Could you check a few things on this model? Use its own coordinates, in mm. A direction names the side the tool comes from. Round coordinates to 2 decimals unless told otherwise and drop trailing zeros. Write each loop counter-clockwise with the first axis right and the second up, starting at its lowest first coordinate (ties: lowest second). Pieces come first, ordered by that corner, then holes. Notation, with made-up numbers: (34, -25.75) -> (73, -25.75) arc R14 cw to (73, -13.75) -> close; hole circle Ø3 at (24, 52.25). An arc over 180 degrees is marked (long way). One line per question, with ' | ' between items. Start each with the question number.
1. For faces 4 (the flat face through (16, -3, 10)), 5 (the flat face through (0, 0, -8)), 6 (the flat face through (0, 0, 5)), 7 (the cylindrical face through (-0.29, 2.23, -3.94)), which set-ups out of +Z, -Z, +X, -X, +Y, -Y let a thin tool reach every point of the face, with its end or its side?
2. If I drill on line 1 along Y through (x, z) = (21.75, 25); line 2 along X through (y, z) = (-4, 27); line 3 along Z through (x, y) = (23.5, -1), over which ranges is the centre line in solid material (lowest first)? Write a range as [from, to].
3. Imagine slicing it at C-C, the plane x = 0. List the corners of the cut face in (y, z) for me, and give its area (3 significant figures).
4. Imagine slicing it at B-B, the plane z = 25. List the corners of the cut face in (x, y) for me.
5. Imagine slicing it at A-A, the plane y = 0. List the corners of the cut face in (x, z) for me.
6. For pin 1 Ø1.5 at (x, z) = (9, 8.5) entering from -Y; pin 2 Ø1.5 at (x, y) = (9.5, 0.5) entering from +Z; pin 3 Ø6.5 at (x, z) = (19, 15) entering from +Y; pin 4 Ø4 at (x, z) = (20.5, 22.5) entering from -Y, each with a flat end and sliding along its axis, tell me the tip position at first contact or that it passes through.
7. Imagine slicing it at D-D, the plane z = -1. List the corners of the cut face in (x, y) for me, and give its area (3 significant figures).
8. Thinking about a two-plate mould opening in Z: for faces 1 (the cylindrical face through (23, 0, 30)), 2 (the flat face through (15, 3, 9)), 3 (the cylindrical face through (22.5, 0.1, 22.5)), which applies, released by +Z, released by -Z, zero draft, split by the parting line, or undercut?
from build123d import *

# Parameters (mm, degrees)
SKETCH_2_R           = 5
EXTRUDE_3_DEPTH      = 5
EXTRUDE_4_DEPTH      = 3
EXTRUDE_4_DEPTH_BACK = 3
SKETCH_3_3_W         = 5
SKETCH_3_3_H         = 5
SKETCH_4_W           = 5
SKETCH_4_H           = 6
EXTRUDE_5_DEPTH      = 3
SKETCH_5_W           = 5
SKETCH_5_H           = 6
EXTRUDE_6_DEPTH      = 3
SKETCH_6_R           = 2.5
CUT_EXTRUDE_1_DEPTH  = 5
EXTRUDE_START        = -5
SKETCH_7_R           = 2.25
EXTRUDE_7_DEPTH      = 8


with BuildPart() as part:
    # Sketch 2 → Extrude 3 (new body)
    with BuildSketch(Plane.XY):
        Circle(SKETCH_2_R)
    extrude(amount=EXTRUDE_3_DEPTH)



with BuildPart() as body_2:
    # Sketch 3 → Extrude 4 (new, two sides: drawn at the far end of the back side and taken through both)
    with BuildSketch(Plane(origin=(0, 0, 0), x_dir=(1, 0, 0), z_dir=(0, 1, 0)).offset(-EXTRUDE_4_DEPTH_BACK)):
        with BuildLine():
            ThreePointArc((5, 0), (18.027756377, -6.972243623), (25, -20))
            Line((25, -20), (20, -20))
            ThreePointArc((20, -20), (14.577379737, -10.422620263), (5, -5))
            Line((5, -5), (5, 0))
        make_face()
    extrude(amount=EXTRUDE_4_DEPTH + EXTRUDE_4_DEPTH_BACK)



with BuildPart() as body_3:
    # Sketch 3_3 → Revolve 1 (revolve)
    with BuildSketch(Plane(origin=(0, 0, 0), x_dir=(1, 0, 0), z_dir=(0, 1, 0)), mode=Mode.PRIVATE) as revolve_1_sk:
        with Locations((22.5, -22.5)):
            Rectangle(SKETCH_3_3_W, SKETCH_3_3_H)
    revolve(revolve_1_sk.sketch.rotate(Axis((0, 0, 25), (1, 0, 0)), 180), axis=Axis((0, 0, 25), (1, 0, 0)))


with BuildPart() as body_2_1:
    add(body_2.part)

    add(body_3.part)  # Extrude 5 merges body 3
    # Sketch 4 → Extrude 5 (add)
    with BuildSketch(Plane.XY.offset(20)):
        with Locations((22.5, 0)):
            Rectangle(SKETCH_4_W, SKETCH_4_H)
    extrude(amount=EXTRUDE_5_DEPTH)


with BuildPart() as part_1:
    add(part.part)

    add(body_2_1.part)  # Extrude 6 merges body 2
    # Sketch 5 → Extrude 6 (add)
    with BuildSketch(Plane.ZY.offset(-5)):
        with Locations((2.5, 0)):
            Rectangle(SKETCH_5_W, SKETCH_5_H)
    extrude(amount=EXTRUDE_6_DEPTH)

    # Sketch 6 → Cut-Extrude 1 (cut)
    with BuildSketch(Plane.ZY.offset(-20)):
        with Locations((25, 0)):
            Circle(SKETCH_6_R)
    extrude(amount=-CUT_EXTRUDE_1_DEPTH, mode=Mode.SUBTRACT)

    # Sketch 7 → Extrude 7 (add)
    with BuildSketch(Plane.XY.offset(5).offset(EXTRUDE_START)):
        Circle(SKETCH_7_R)
    extrude(amount=-EXTRUDE_7_DEPTH)


solid = part_1.part
Geometry results:
1) face 4: -Z, +X, -Y | face 5: -Z, +X, -X, +Y, -Y | face 6: +Z, -X, +Y, -Y | face 7: -Z
2) line 1: y = [-5, -2.5], [2.5, 5] | line 2: x = [20, 25] | line 3: z = [15.11, 22.71], [27.29, 29.9]
3) outline: (-5, 0) -> (-2.25, 0) -> (-2.25, -8) -> (2.25, -8) -> (2.25, 0) -> (5, 0) -> (5, 5) -> (-5, 5) -> close | area: 86.0 mm2
4) outline: (20, -5) -> (25, -5) -> (25, -2.5) -> (20, -2.5) -> close; (20, 2.5) -> (25, 2.5) -> (25, 5) -> (20, 5) -> close
5) outline: (-5, 0) -> (-2.25, 0) -> (-2.25, -8) -> (2.25, -8) -> (2.25, 0) -> (5, 0) arc R25.5 ccw to (25, 20) -> (25, 22.5) -> (20, 22.5) -> (20, 20) arc R20.62 cw to (5, 5) -> (-5, 5) -> close; (20, 27.5) -> (25, 27.5) -> (25, 30) -> (20, 30) -> close
6) pin 1: passes through | pin 2: stops at z = 7.11 | pin 3: stops at y = 3 | pin 4: stops at y = -4.97
7) outline: circle Ø4.5 at (0, 0) | area: 15.9 mm2
8) face 1: split by the parting line | face 2: zero draft | face 3: undercut
